Work out the finished part from the listing and answer in its coordinate system (mm). A direction names the side the tool comes from. Round coordinates to 2 decimals unless told otherwise and drop trailing zeros. Order: outer loops, then holes, each group sorted by start corner. A loop starts at its lowest first (then second) coordinate and runs counter-clockwise, first axis right, second up. Notation, with made-up numbers: M 46,6 L 58,6 A19 ccw 58,17 Z; hole C -6,88 d10. An arc over 180 degrees is marked long. Return JSON: item names as keys, results as strings.
from build123d import *

# Parameters (mm, degrees)
BOSS_EXTRUDE1_DEPTH = 18
BOSS_EXTRUDE3_DEPTH = 20


with BuildPart() as part:
    # Sketch3 → Boss-Extrude1 (new body)
    with BuildSketch(Plane(origin=(0, 0, 0), x_dir=(1, 0, 0), z_dir=(0, 1, 0))):
        with BuildLine():
            Line((0, 0), (-930, 0))
            Line((-930, 0), (-930, 540))
            ThreePointArc((-930, 540), (-883.13708499, 653.13708499), (-770, 700))
            add(Edge.make_bspline(
                [(-770, 700), (-664.69635322, 719.084597111), (-573.996492447, 783.951968622), (-465, 789.509158613)],
                knots=[0, 0, 0, 0, 1, 1, 1, 1], degree=3))
            add(Edge.make_bspline(
                [(-160, 700), (-265.30364678, 719.084597111), (-356.003507553, 783.951968622), (-465, 789.509158613)],
                knots=[0, 0, 0, 0, 1, 1, 1, 1], degree=3))
            ThreePointArc((-160, 700), (-46.86291501, 653.13708499), (0, 540))
            Line((0, 540), (0, 0))
        make_face()
        with BuildLine():
            Line((-20, 150), (-38, 150))
            ThreePointArc((-38, 150), (-44.35, 156.35), (-38, 162.7))
            Line((-38, 162.7), (-38, 197.3))
            ThreePointArc((-38, 197.3), (-44.35, 203.65), (-38, 210))
            Line((-38, 210), (-20, 210))
            ThreePointArc((-20, 210), (-13.65, 203.65), (-20, 197.3))
            Line((-20, 197.3), (-20, 162.7))
            ThreePointArc((-20, 162.7), (-13.65, 156.35), (-20, 150))
        make_face(mode=Mode.SUBTRACT)
        with BuildLine():
            Line((-910, 450), (-892, 450))
            ThreePointArc((-892, 450), (-885.65, 456.35), (-892, 462.7))
            Line((-892, 462.7), (-892, 497.3))
            ThreePointArc((-892, 497.3), (-885.65, 503.65), (-892, 510))
            Line((-892, 510), (-910, 510))
            ThreePointArc((-910, 510), (-916.35, 503.65), (-910, 497.3))
            Line((-910, 497.3), (-910, 462.7))
            ThreePointArc((-910, 462.7), (-916.35, 456.35), (-910, 450))
        make_face(mode=Mode.SUBTRACT)
        with BuildLine():
            Line((-910, 300), (-892, 300))
            ThreePointArc((-892, 300), (-885.65, 306.35), (-892, 312.7))
            Line((-892, 312.7), (-892, 347.3))
            ThreePointArc((-892, 347.3), (-885.65, 353.65), (-892, 360))
            Line((-892, 360), (-910, 360))
            ThreePointArc((-910, 360), (-916.35, 353.65), (-910, 347.3))
            Line((-910, 347.3), (-910, 312.7))
            ThreePointArc((-910, 312.7), (-916.35, 306.35), (-910, 300))
        make_face(mode=Mode.SUBTRACT)
        with BuildLine():
            Line((-910, 150), (-892, 150))
            ThreePointArc((-892, 150), (-885.65, 156.35), (-892, 162.7))
            Line((-892, 162.7), (-892, 197.3))
            ThreePointArc((-892, 197.3), (-885.65, 203.65), (-892, 210))
            Line((-892, 210), (-910, 210))
            ThreePointArc((-910, 210), (-916.35, 203.65), (-910, 197.3))
            Line((-910, 197.3), (-910, 162.7))
            ThreePointArc((-910, 162.7), (-916.35, 156.35), (-910, 150))
        make_face(mode=Mode.SUBTRACT)
        with BuildLine():
            Line((-38, 312.7), (-38, 347.3))
            ThreePointArc((-38, 347.3), (-44.35, 353.65), (-38, 360))
            Line((-38, 360), (-20, 360))
            ThreePointArc((-20, 360), (-13.65, 353.65), (-20, 347.3))
            Line((-20, 347.3), (-20, 312.7))
            ThreePointArc((-20, 312.7), (-13.65, 306.35), (-20, 300))
            Line((-20, 300), (-38, 300))
            ThreePointArc((-38, 300), (-44.35, 306.35), (-38, 312.7))
        make_face(mode=Mode.SUBTRACT)
        with BuildLine():
            Line((-20, 450), (-38, 450))
            ThreePointArc((-38, 450), (-44.35, 456.35), (-38, 462.7))
            Line((-38, 462.7), (-38, 497.3))
            ThreePointArc((-38, 497.3), (-44.35, 503.65), (-38, 510))
            Line((-38, 510), (-20, 510))
            ThreePointArc((-20, 510), (-13.65, 503.65), (-20, 497.3))
            Line((-20, 497.3), (-20, 462.7))
            ThreePointArc((-20, 462.7), (-13.65, 456.35), (-20, 450))
        make_face(mode=Mode.SUBTRACT)
    extrude(amount=BOSS_EXTRUDE1_DEPTH)

    # Sketch4 → Boss-Extrude3 (add)
    with BuildSketch(Plane(origin=(0, 18, 0), x_dir=(1, 0, 0), z_dir=(0, 1, 0))):
        with BuildLine():
            Line((-379.222882365, 485.717294758), (-382.737003031, 490.02028309))
            Line((-382.737003031, 490.02028309), (-373.95352551, 497.187167352))
            Line((-373.95352551, 497.187167352), (-370.170166428, 492.550417512))
            ThreePointArc((-370.170166428, 492.550417512), (-315.881947929, 625.006423951), (-397.403737413, 742.675460443))
            Line((-397.403737413, 742.675460443), (-399.595153576, 737.371427218))
            Line((-399.595153576, 737.371427218), (-410.077786811, 741.702435514))
            Line((-410.077786811, 741.702435514), (-407.722392765, 747.403355536))
            ThreePointArc((-407.722392765, 747.403355536), (-553.118476248, 730.158011216), (-614.556786971, 597.256705849))
            Line((-614.556786971, 597.256705849), (-609.305354492, 598.063637084))
            Line((-609.305354492, 598.063637084), (-607.58398502, 586.861126686))
            Line((-607.58398502, 586.861126686), (-613.25925572, 585.989068783))
            ThreePointArc((-613.25925572, 585.989068783), (-524.072934254, 470.893038587), (-379.222882365, 485.717294758))
        make_face()
        with BuildLine():
            Line((-605.954754503, 598.578487803), (-604.233385032, 587.375977405))
            Line((-604.233385032, 587.375977405), (-597.029293803, 588.482952741))
            Line((-597.029293803, 588.482952741), (-568.840566092, 552.629818575))
            ThreePointArc((-568.840566092, 552.629818575), (-566.026361545, 550.558864621), (-562.547777239, 550.230156949))
            Line((-562.547777239, 550.230156949), (-544.012184687, 553.5242975))
            ThreePointArc((-544.012184687, 553.5242975), (-540.701764813, 555.173597747), (-538.813218815, 558.353607977))
            add(Edge.make_bspline(
                [(-538.813218815, 558.353607977), (-534.297460402, 576.070334999), (-503.019078365, 584.719773706), (-464.685769523, 573.113632357), (-440.044169756, 551.361798965), (-435.372177088, 522.801108934), (-465.299141833, 494.166605222), (-498.623668355, 508.836515007), (-515.396755845, 517.710933859)],
                knots=[0.009911477, 0.009911477, 0.009911477, 0.009911477, 0.210711156, 0.384962621, 0.515680366, 0.61771746, 0.71863394, 0.985505172, 0.985505172, 0.985505172, 0.985505172], degree=3))
            ThreePointArc((-515.396755845, 517.710933859), (-517.304141637, 518.368440775), (-519.321159046, 518.414011368))
            Line((-519.321159046, 518.414011368), (-528.660749273, 517.173060959))
            ThreePointArc((-528.660749273, 517.173060959), (-533.640663746, 513.638476733), (-533.538280042, 507.532549172))
            Line((-533.538280042, 507.532549172), (-521.15107554, 484.961134511))
            ThreePointArc((-521.15107554, 484.961134511), (-518.367019202, 482.26890411), (-514.548775713, 481.620759927))
            Line((-514.548775713, 481.620759927), (-389.451748889, 498.242389225))
            Line((-389.451748889, 498.242389225), (-385.513228418, 493.419729662))
            Line((-385.513228418, 493.419729662), (-376.731376811, 500.591602748))
            Line((-376.731376811, 500.591602748), (-380.563507134, 505.28812488))
            Line((-380.563507134, 505.28812488), (-365.655848241, 541.370143173))
            ThreePointArc((-365.655848241, 541.370143173), (-365.165238954, 544.139540747), (-365.881745133, 546.85926119))
            Line((-365.881745133, 546.85926119), (-372.699432744, 560.146905814))
            ThreePointArc((-372.699432744, 560.146905814), (-375.904525506, 563.158238505), (-380.291797246, 563.462525982))
            add(Edge.make_bspline(
                [(-380.291797246, 563.462525982), (-389.62136338, 560.847813387), (-407.34030176, 567.487642274), (-419.84509917, 588.039259046), (-426.364337105, 610.176048947), (-426.75390148, 634.572716458), (-418.374308101, 656.599818062), (-401.385797189, 668.865586287), (-379.856576304, 666.13746701), (-359.465829462, 641.758569228), (-355.228193135, 617.579148091), (-354.680419376, 601.80580369)],
                knots=[0.0061934, 0.0061934, 0.0061934, 0.0061934, 0.129362399, 0.215046737, 0.307702519, 0.422372662, 0.521838861, 0.597629821, 0.671660902, 0.77578766, 0.978099053, 0.978099053, 0.978099053, 0.978099053], degree=3))
            ThreePointArc((-354.680419376, 601.80580369), (-354.473650835, 600.385356434), (-353.962320397, 599.044101492))
            Line((-353.962320397, 599.044101492), (-351.783279864, 594.797160611))
            ThreePointArc((-351.783279864, 594.797160611), (-345.688613875, 591.244158092), (-339.906500201, 595.285932686))
            Line((-339.906500201, 595.285932686), (-329.168313442, 621.276294679))
            ThreePointArc((-329.168313442, 621.276294679), (-328.718783675, 624.556387197), (-329.931425401, 627.637066339))
            Line((-329.931425401, 627.637066339), (-403.370553681, 728.233570185))
            Line((-403.370553681, 728.233570185), (-401.527937134, 732.693380033))
            Line((-401.527937134, 732.693380033), (-412.01057037, 737.024388329))
            Line((-412.01057037, 737.024388329), (-413.853186916, 732.564578481))
            Line((-413.853186916, 732.564578481), (-453.198107375, 727.394628039))
            ThreePointArc((-453.198107375, 727.394628039), (-456.332644817, 726.096116164), (-458.396434076, 723.403119327))
            Line((-458.396434076, 723.403119327), (-465.579522616, 706.017402764))
            ThreePointArc((-465.579522616, 706.017402764), (-465.917084215, 702.084917604), (-463.932980801, 698.672920972))
            add(Edge.make_bspline(
                [(-463.932980801, 698.672920972), (-456.316914214, 691.747841587), (-451.453700795, 670.847901054), (-468.128106478, 647.707017887), (-487.409129401, 628.723458004), (-512.02899646, 620.595846866), (-535.731034887, 620.753825005), (-548.494456823, 635.551717206), (-553.67838325, 668.726301345), (-523.496250086, 689.825139347), (-509.375871044, 699.500113635)],
                knots=[0.010513604, 0.010513604, 0.010513604, 0.010513604, 0.140440996, 0.245214617, 0.361326435, 0.482761337, 0.571282501, 0.643749642, 0.712105448, 0.981383935, 0.981383935, 0.981383935, 0.981383935], degree=3))
            ThreePointArc((-509.375871044, 699.500113635), (-507.989430568, 700.779548939), (-507.02535105, 702.401190876))
            Line((-507.02535105, 702.401190876), (-503.168441841, 711.736329924))
            ThreePointArc((-503.168441841, 711.736329924), (-503.864230082, 718.003151755), (-509.526748851, 720.776788059))
            Line((-509.526748851, 720.776788059), (-545.744632169, 719.076899224))
            ThreePointArc((-545.744632169, 719.076899224), (-549.204312297, 717.892164096), (-551.489001713, 715.036787031))
            Line((-551.489001713, 715.036787031), (-599.174501495, 599.620336472))
            Line((-599.174501495, 599.620336472), (-605.954754503, 598.578487803))
        make_face(mode=Mode.SUBTRACT)
    extrude(amount=BOSS_EXTRUDE3_DEPTH)


solid = part.part
Item 1: The mould has two halves that part along Z. Classify faces 4 (the flat face through (-458, 18, -313)), 5 (the flat face through (-373.214, 27.86, -523.077)), 6 (the cylindrical face through (-315.67, 27.86, -622.93)): pulls with the +Z half, pulls with the -Z half, needs draft (parallel to the pull), parting line crosses it, or undercut.
Output:
{"face 4": "needs draft", "face 5": "undercut", "face 6": "parting line crosses it"}
Item 2: Consider line 1 along X through (y, z) = (12.5, -333); line 2 along Z through (x, y) = (-419.5, 30); line 3 along Z through (x, y) = (-446, 21.5). Determine where each line is inside the solid, lowest interval first. Write a range as [from, to].
Output:
{"line 1": "x = [-930, -910], [-892, -38], [-20, 0]", "line 2": "z = [-751.7, -731.82], [-651.04, -589.56], [-494.25, -465.84]", "line 3": "z = [-757.56, -728.34], [-554.45, -513.67], [-490.73, -459.98]"}
Item 3: Which of the six approach directions +Z, -Z, +X, -X, +Y, -Y give full straight-line access (tool end or side, diameter ignored) to faces 1 (the cylindrical face through (-526.023, 27.86, -471.745)), 2 (the flat face through (-527.38, 27.86, -719.94)), 3 (the flat face through (-500, 38, -578))?
Output:
{"face 1": "+Z, +Y", "face 2": "+Y", "face 3": "+Z, -Z, +X, -X, +Y"}
Item 4: Each of these flat-tipped pins is pushed along its axis until it touches: pin 1 (5.5 mm diameter, centred on x = -28, y = 12.5, fed in from -Z); pin 2 (3 mm diameter, centred on x = -395, y = 5, fed in from -Z); pin 3 (5.5 mm diameter, centred on x = -904, y = 11.5, fed in from -Z); pin 4 (4 mm diameter, centred on x = -809, y = 21, fed in from +Z). Where does it stop, or does it pass through?
Output:
{"pin 1": "stops at z = -634.31", "pin 2": "stops at z = -778.64", "pin 3": "stops at z = -631.51", "pin 4": "passes through"}
Item 5: Find section A-A (z = -249). Determine the outline of the cut face in (x, y), plus the area to 3 significant figures.
Output:
{"outline": "M -930,0 L 0,0 L 0,18 L -930,18 Z", "area": "16,700 mm^2"}
